Geometry check sheet. Reference: the model listing, model coordinates, mm. Round coordinates to 2 decimals unless told otherwise and drop trailing zeros. Write each loop counter-clockwise with the first axis right and the second up, starting at its lowest first coordinate (ties: lowest second). Pieces come first, ordered by that corner, then holes. Notation, with made-up numbers: (42.25, 42) - (101.25, 42) arc R34 cw to (101.25, 72) - close; hole circle Ø7 at (9.5, 4.5). An arc over 180 degrees is marked (long way). Return JSON: item names as keys, results as strings. Group by question number.
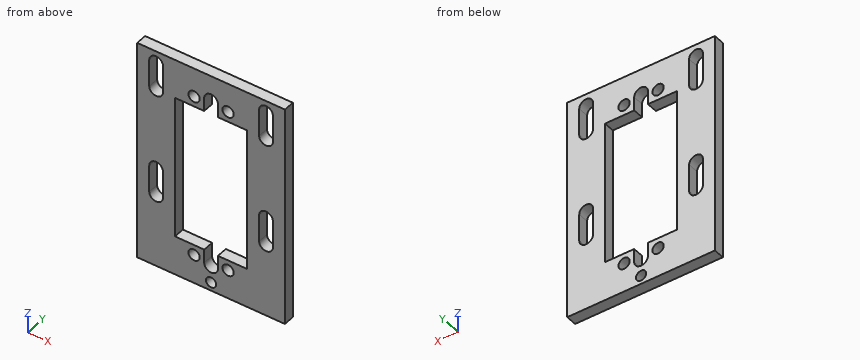
from build123d import *

# Parameters (mm, degrees)
SKETCH1_W           = 43
SKETCH1_H           = 65
SKETCH1_R           = 1.65
BOSS_EXTRUDE1_DEPTH = 3.175
CUT_EXTRUDE1_DEPTH  = 3.175
SKETCH4_R           = 1.5
CUT_EXTRUDE2_DEPTH  = 10


with BuildPart() as part:
    # Sketch1 → Boss-Extrude1 (new body)
    with BuildSketch(Plane(origin=(0, 0, 0), x_dir=(1, 0, 0), z_dir=(0, 1, 0))):
        Rectangle(SKETCH1_W, SKETCH1_H)
        with Locations(Location((-4.95, -24, 0), (0, 0, 270))):
            Circle(SKETCH1_R, mode=Mode.SUBTRACT)
        with BuildLine():
            Line((-10.5, 21), (-2, 21))
            Line((-2, 21), (-2, 24))
            Line((-2, 24), (-2, 25))
            ThreePointArc((-2, 25), (0, 27), (2, 25))
            Line((2, 25), (2, 24))
            Line((2, 24), (2, 21))
            Line((2, 21), (10.5, 21))
            Line((10.5, 21), (10.5, 0))
            Line((10.5, 0), (10.5, -21))
            Line((10.5, -21), (2, -21))
            Line((2, -21), (2, -24))
            Line((2, -24), (2, -25))
            ThreePointArc((2, -25), (0, -27), (-2, -25))
            Line((-2, -25), (-2, -24))
            Line((-2, -24), (-2, -21))
            Line((-2, -21), (-10.5, -21))
            Line((-10.5, -21), (-10.5, 0))
            Line((-10.5, 0), (-10.5, 21))
        make_face(mode=Mode.SUBTRACT)
        with BuildLine():
            ThreePointArc((6.6, -24), (4.95, -25.65), (3.3, -24))
            ThreePointArc((3.3, -24), (4.95, -22.35), (6.6, -24))
        make_face(mode=Mode.SUBTRACT)
        with Locations(Location((-4.95, 24, 0), (0, 0, 270))):
            Circle(SKETCH1_R, mode=Mode.SUBTRACT)
        with BuildLine():
            ThreePointArc((6.6, 24), (4.95, 22.35), (3.3, 24))
            ThreePointArc((3.3, 24), (4.95, 25.65), (6.6, 24))
        make_face(mode=Mode.SUBTRACT)
    extrude(amount=BOSS_EXTRUDE1_DEPTH)

    # Sketch3 → Cut-Extrude1 (cut)
    with BuildSketch(Plane(origin=(0, 3.175, 0), x_dir=(1, 0, 0), z_dir=(0, 1, 0))):
        with BuildLine():
            Line((-14, -21), (-14, -29))
            ThreePointArc((-14, -29), (-16, -31), (-18, -29))
            Line((-18, -29), (-18, -21))
            ThreePointArc((-18, -21), (-16, -19), (-14, -21))
        make_face()
        with BuildLine():
            Line((14, -21), (14, -29))
            ThreePointArc((14, -29), (16, -31), (18, -29))
            Line((18, -29), (18, -21))
            ThreePointArc((18, -21), (16, -19), (14, -21))
        make_face()
        with BuildLine():
            Line((-14, 11), (-14, 3))
            ThreePointArc((-14, 3), (-16, 1), (-18, 3))
            Line((-18, 3), (-18, 11))
            ThreePointArc((-18, 11), (-16, 13), (-14, 11))
        make_face()
        with BuildLine():
            Line((14, 11), (14, 3))
            ThreePointArc((14, 3), (16, 1), (18, 3))
            Line((18, 3), (18, 11))
            ThreePointArc((18, 11), (16, 13), (14, 11))
        make_face()
    extrude(amount=-CUT_EXTRUDE1_DEPTH, mode=Mode.SUBTRACT)

    # Sketch4 → Cut-Extrude2 (cut)
    with BuildSketch(Plane(origin=(0, 3.175, 0), x_dir=(1, 0, 0), z_dir=(0, 1, 0))):
        with Locations(Location((0, 30, 0), (0, 0, 270))):
            Circle(SKETCH4_R)
    extrude(amount=-CUT_EXTRUDE2_DEPTH, mode=Mode.SUBTRACT)


solid = part.part
1. Material ranges on line 1 along Z through (x, y) = (5, 0.3); line 2 along X through (y, z) = (2.95, 21.5); line 3 along X through (y, z) = (1.5, 24), recorded low to high.
2. Depth check by flat-ended pin: pin 1 Ø6 at (x, z) = (10.5, -3) entering from -Y; pin 2 Ø2 at (x, z) = (1, 18.5) entering from +Y. Enter the tip coordinate at first touch or a pass-through.
3. Section check B-B (x = -16). Enter the section's corners in (y, z) (3 decimals).
4. Section check A-A (z = 24). Enter the section's corners in (x, y) (3 decimals).
5. Section check C-C (z = -14). Enter the section's corners in (x, y) (3 decimals), and give its area (4 significant figures).
6. Section check D-D (y = 1.5). State how many separate pieces and enclosed holes the cut face has, and give its area (3 significant figures).
Result sheet:
{
 "1": {"line 1": "z = -32.5 to -25.65, -22.35 to -21, 21 to 22.35, 25.65 to 32.5", "line 2": "x = -21.5 to -18, -14 to -2, 2 to 14, 18 to 21.5", "line 3": "x = -21.5 to -18, -14 to -6.6, -3.3 to -2, 2 to 3.3, 6.6 to 14, 18 to 21.5"},
 "2": {"pin 1": "stops at y = 0", "pin 2": "passes through"},
 "3": {"outline": "(0, -32.5) - (3.175, -32.5) - (3.175, -13) - (0, -13) - close; (0, -1) - (3.175, -1) - (3.175, 19) - (0, 19) - close; (0, 31) - (3.175, 31) - (3.175, 32.5) - (0, 32.5) - close"},
 "4": {"outline": "(-21.5, 0) - (-18, 0) - (-18, 3.175) - (-21.5, 3.175) - close; (-14, 0) - (-6.6, 0) - (-6.6, 3.175) - (-14, 3.175) - close; (-3.3, 0) - (-2, 0) - (-2, 3.175) - (-3.3, 3.175) - close; (2, 0) - (3.3, 0) - (3.3, 3.175) - (2, 3.175) - close; (6.6, 0) - (14, 0) - (14, 3.175) - (6.6, 3.175) - close; (18, 0) - (21.5, 0) - (21.5, 3.175) - (18, 3.175) - close"},
 "5": {"outline": "(-21.5, 0) - (-10.5, 0) - (-10.5, 3.175) - (-21.5, 3.175) - close; (10.5, 0) - (21.5, 0) - (21.5, 3.175) - (10.5, 3.175) - close", "area": "69.85 mm²"},
 "6": {"separate pieces": "1", "enclosed holes": "10", "area": "1,650 mm²"}
}
